Check sheet for the modelled part. Datum: model origin and axes. Units: mm. A direction names the side the tool comes from. Round coordinates to 2 decimals unless told otherwise and drop trailing zeros. Order: outer loops, then holes, each group sorted by start corner. A loop starts at its lowest first (then second) coordinate and runs counter-clockwise, first axis right, second up. Notation, with made-up numbers: (10, 72) -> (61, 72) arc R12 cw to (61, 86) -> close; hole circle Ø2 at (22, 70.25). An arc over 180 degrees is marked (long way). Use CSV: the item, a comma, the result in double quotes.
```python
from build123d import *

# Parameters (mm, degrees)
F0_R     = 12.7
F0_R_2   = 5.3594
F1_DEPTH = 12.7
F2_DEPTH = 19.05
F3_R     = 9.525
F4_DEPTH = 50.8


with BuildPart() as f1:
    # F0 (on Front) → F1 (new body)
    with BuildSketch(Plane.XZ):
        Circle(F0_R)
        Circle(F0_R_2, mode=Mode.SUBTRACT)
        Circle(F0_R_2)
    extrude(amount=F1_DEPTH)

    # F0 (on Front) → F2 (join)
    with BuildSketch(Plane.XZ):
        Circle(F0_R_2)
    extrude(amount=-F2_DEPTH)

    # F3 (on face) → F4 (join)
    with BuildSketch(Plane.XZ.offset(12.7)):
        Circle(F3_R)
    extrude(amount=F4_DEPTH)


solid = f1.part
```
Q1. Go/stop test with flat-tipped pins: pin 1 (12 mm diameter, centred on y = -46, z = -4, fed in from -X) (3 decimals); pin 2 (10 mm diameter, centred on x = -8.5, z = 7, fed in from +Y); pin 3 (5 mm diameter, centred on x = 9.5, y = -11.5, fed in from +Z). Record where each tip stops, or that it passes through.
Result sheet:
pin 1,"stops at x = -9.525"
pin 2,"stops at y = 0"
pin 3,"stops at z = 10.6"
Q2. Sectioned sample at D-D, the plane z = 8. Enter the section's corners in (x, y).
Result sheet:
outline,"(-9.86, -12.7) -> (-5.17, -12.7) -> (-5.17, -63.5) -> (5.17, -63.5) -> (5.17, -12.7) -> (9.86, -12.7) -> (9.86, 0) -> (-9.86, 0) -> close"
Q3. Sectioned sample at B-B, the plane x = 0. Enter the section's corners in (y, z) (3 decimals), then the cut area to 3 significant figures.
Result sheet:
outline,"(-63.5, -9.525) -> (-12.7, -9.525) -> (-12.7, -12.7) -> (0, -12.7) -> (0, -5.359) -> (19.05, -5.359) -> (19.05, 5.359) -> (0, 5.359) -> (0, 12.7) -> (-12.7, 12.7) -> (-12.7, 9.525) -> (-63.5, 9.525) -> close"
area,"1,490 mm^2"
Q4. Access from +Z, -Z, +X, -X, +Y, -Y to the whole of each face (thin tool, end or side, straight path). Record for faces 1 (the face through (5, -12.7, 9)), 2 (the face through (5, 0, -3)), 3 (the face through (0, -63.5, 0)).
Result sheet:
face 1,"-Y"
face 2,"+Y"
face 3,"+Z, -Z, +X, -X, -Y"
Q5. Sectioned sample at C-C, the plane y = -8.5. Enter the section's corners in (x, z).
Result sheet:
outline,"circle Ø25.4 at (0, 0)"
Q6. Sectioned sample at A-A, the plane z = 0. Enter the section's corners in (x, y) (3 decimals).
Result sheet:
outline,"(-12.7, -12.7) -> (-9.525, -12.7) -> (-9.525, -63.5) -> (9.525, -63.5) -> (9.525, -12.7) -> (12.7, -12.7) -> (12.7, 0) -> (5.359, 0) -> (5.359, 19.05) -> (-5.359, 19.05) -> (-5.359, 0) -> (-12.7, 0) -> close"
Q7. Scan lines: L1, parallel to Y at x = 1, z = 7.25; L2, parallel to Y at x = 11, z = -6.25; L3, parallel to X at y = -14, z = 0.25. Record each from-to range of solid material in increasing order.
Result sheet:
L1,"y = -63.5 to 0"
L2,"y = -12.7 to 0"
L3,"x = -9.52 to 9.52"
